Read the model definition and answer for the solid it produces. Units are mm, in the model's axes. Round coordinates to 2 decimals unless told otherwise and drop trailing zeros. Write each loop counter-clockwise with the first axis right and the second up, starting at its lowest first coordinate (ties: lowest second). Pieces come first, ordered by that corner, then holes. Notation, with made-up numbers: (77, 62) - (111, 62) arc R27 cw to (111, 89) - close; hole circle Ø3 at (-6, 20). An arc over 180 degrees is marked (long way). Answer as CSV lines item,"result". Start each with the question number.
1) Find section A-A on y = -24.75. Determine the outline of the cut face in (x, z), then the cut area to 3 significant figures.
2) Consider line 1 along Y through (x, z) = (0, 2.2); line 2 along X through (y, z) = (25.5, 3.3); line 3 along Y through (x, z) = (-0.5, 0.2). Determine where each line is inside the solid, lowest interval first.
3) This flat-tipped pin is pushed along its axis until it touches: pin 1 (4 mm diameter, centred on x = 5, y = -24.75, fed in from +Z). Where does it stop, or does it pass through?
4) Find section B-B on x = 0. Determine the outline of the cut face in (y, z), then the cut area to 3 significant figures.
5) Find section C-C on y = 6.5. Determine the outline of the cut face in (x, z).
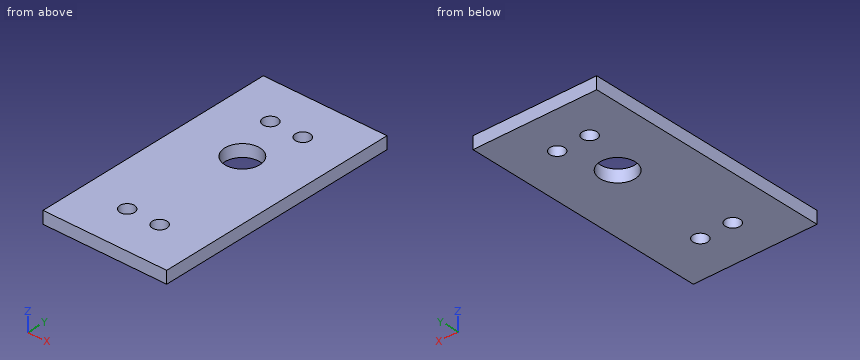
from build123d import *

# Parameters (mm, degrees)
SKETCH1_W            = 38.1
SKETCH1_H            = 76.2
BOSS_EXTRUDE1_DEPTH  = 3.81
M4_CLEARANCE_HOLE1_D = 4.5
CUT_EXTRUDE1_REACH   = 44.767
SKETCH5_R            = 5.3975


with BuildPart() as part:
    # Sketch1 → Boss-Extrude1 (new body)
    with BuildSketch(Plane.XY):
        Rectangle(SKETCH1_W, SKETCH1_H)
    extrude(amount=BOSS_EXTRUDE1_DEPTH)

    # M4 Clearance Hole1 (through all)
    with Locations(Plane.XY.offset(3.81)):
        with Locations((-5, 24.75), (5, 24.75), (-5, -24.75), (5, -24.75)):
            Hole(M4_CLEARANCE_HOLE1_D / 2)

    # Sketch5 → Cut-Extrude1 (cut, up to next)
    with BuildSketch(Plane.XY.offset(3.81), mode=Mode.PRIVATE) as cut_extrude1_sk1:
        with Locations((0, 9.464)):
            Circle(SKETCH5_R)
    cut_extrude1_tool1 = extrude(cut_extrude1_sk1.sketch, amount=-CUT_EXTRUDE1_REACH, mode=Mode.PRIVATE) & part.part
    add(cut_extrude1_tool1.solids().sort_by_distance((0, 9.464, 3.81))[0], mode=Mode.SUBTRACT)


solid = part.part
Check values:
1,outline,"(-19.05, 0) - (-7.25, 0) - (-7.25, 3.81) - (-19.05, 3.81) - close; (-2.75, 0) - (2.75, 0) - (2.75, 3.81) - (-2.75, 3.81) - close; (7.25, 0) - (19.05, 0) - (19.05, 3.81) - (7.25, 3.81) - close"
1,area,"111 mm^2"
2,line 1,"y = -38.1 to 4.07, 14.86 to 38.1"
2,line 2,"x = -19.05 to -7.12, -2.88 to 2.88, 7.12 to 19.05"
2,line 3,"y = -38.1 to 4.09, 14.84 to 38.1"
3,pin 1,"passes through"
4,outline,"(-38.1, 0) - (4.07, 0) - (4.07, 3.81) - (-38.1, 3.81) - close; (14.86, 0) - (38.1, 0) - (38.1, 3.81) - (14.86, 3.81) - close"
4,area,"249 mm^2"
5,outline,"(-19.05, 0) - (-4.51, 0) - (-4.51, 3.81) - (-19.05, 3.81) - close; (4.51, 0) - (19.05, 0) - (19.05, 3.81) - (4.51, 3.81) - close"
